Verification items for this drawing (mm, ordinates from the low corner). Give positions to 0.01 mm unless a question says otherwise; leave off trailing zeros. Write each loop counter-clockwise with the first axis right and the second up, starting at its lowest first coordinate (ties: lowest second). Pieces come first, ordered by that corner, then holes. Notation, with made-up numbers: (-25.5, -3.5) -> (-16.5, -3.5) arc R19 ccw to (-16.5, 32.5) -> close; hole circle Ø10 at (-4, 18.25). An arc over 180 degrees is marked (long way). Answer as a JSON object with one key per item and string values.
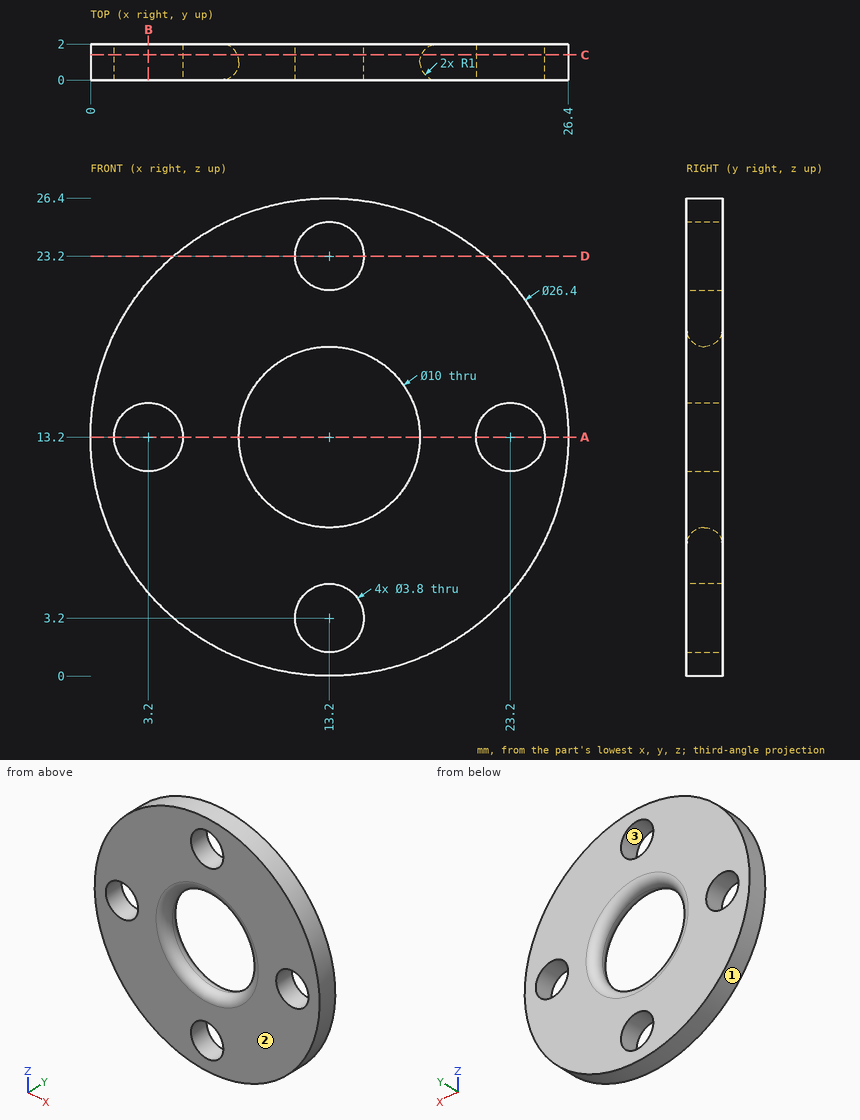
1. Sectioned sample at B-B, the plane x = 3.2. Enter the section's corners in (y, z), plus the area to 3 significant figures.
Determined:
{"outline": "(0, 4.58) -> (2, 4.58) -> (2, 11.3) -> (0, 11.3) -> close; (0, 15.1) -> (2, 15.1) -> (2, 21.82) -> (0, 21.82) -> close", "area": "26.9 mm^2"}
2. Mould release check, pull along Z, two halves, no side actions. Record for the marked faces 1, 2 and 3: released by +Z, released by -Z, zero draft, split by the parting line, or undercut.
Determined:
{"face 1": "split by the parting line", "face 2": "zero draft", "face 3": "undercut"}
3. Sectioned sample at D-D, the plane z = 23.2. Enter the section's corners in (x, y).
Determined:
{"outline": "(4.58, 0) -> (11.3, 0) -> (11.3, 2) -> (4.58, 2) -> close; (15.1, 0) -> (21.82, 0) -> (21.82, 2) -> (15.1, 2) -> close"}
4. Scan lines: L1, parallel to X at y = 0.55, z = 13.5; L2, parallel to X at y = 1.55, z = 16.5; L3, parallel to Z at x = 13, y = 0.75. Record each from-to range of solid material in increasing order. Write a range as [from, to].
Determined:
{"L1": "[0, 1.32], [5.08, 8.1], [18.3, 21.32], [25.08, 26.4]", "L2": "[0.42, 9.23], [17.17, 25.98]", "L3": "[0, 1.31], [5.09, 8.17], [18.23, 21.31], [25.09, 26.4]"}
5. Sectioned sample at C-C, the plane y = 1.4. Enter the section's corners in (x, z).
Determined:
{"outline": "circle Ø26.4 at (13.2, 13.2); hole circle Ø3.8 at (3.2, 13.2); hole circle Ø10.17 at (13.2, 13.2); hole circle Ø3.8 at (13.2, 3.2); hole circle Ø3.8 at (13.2, 23.2); hole circle Ø3.8 at (23.2, 13.2)"}
6. Sectioned sample at A-A, the plane z = 13.2. State how many separate pieces and enclosed holes the cut face has, plus the area to 3 significant figures.
Determined:
{"separate pieces": "4", "enclosed holes": "0", "area": "16.7 mm^2"}
